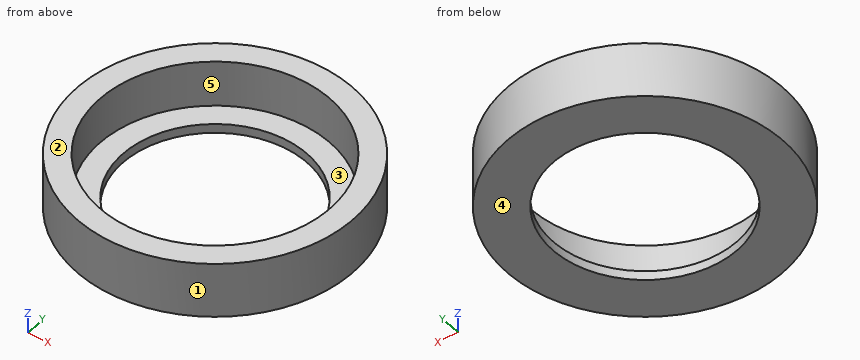
```python
from build123d import *

# Parameters (mm, degrees)
SKETCH_R        = 15
PAD_DEPTH       = 6
SKETCH001_R     = 12.5
POCKET_DEPTH    = 5
SKETCH002_R     = 10
POCKET001_DEPTH = 1.001


with BuildPart() as part:
    # Sketch → Pad (new body)
    with BuildSketch(Plane.XY):
        Circle(SKETCH_R)
    extrude(amount=PAD_DEPTH)

    # Sketch001 (on Face3 of Pad) → Pocket (cut)
    with BuildSketch(Plane.XY.offset(6)):
        Circle(SKETCH001_R)
    extrude(amount=-POCKET_DEPTH, mode=Mode.SUBTRACT)

    # Sketch002 (on Face5 of Pocket) → Pocket001 (cut, through all)
    with BuildSketch(Plane.XY.offset(1)):
        Circle(SKETCH002_R)
    extrude(amount=-POCKET001_DEPTH, mode=Mode.SUBTRACT)


solid = part.part
```
Geometry check sheet. Reference: the model listing, model coordinates, mm. Face numbers are marked on the shaded views. A direction names the side the tool comes from. Coordinates: 2 decimals unless noted, no trailing zeros. Order: outer loops, then holes, each group sorted by start corner. A loop starts at its lowest first (then second) coordinate and runs counter-clockwise, first axis right, second up.
Item 1: Depth check by flat-ended pin: pin 1 (2 mm diameter, centred on y = -5, z = 3, fed in from +X); pin 2 (1 mm diameter, centred on x = 6, z = 1, fed in from +Y); pin 3 (7.5 mm diameter, centred on x = 5.5, y = -5.5, fed in from +Z). Enter the tip coordinate at first touch or a pass-through.
Item 2: Tool access check on the marked faces 4 and 5. Record the directions out of +Z, -Z, +X, -X, +Y, -Y that give a thin tool (end or side, any length) a straight path to the whole face; none if there is none.
Item 3: Section check C-C (z = 0.5). Enter the section's corners in (x, y).
Item 4: Section check A-A (x = 0). Enter the section's corners in (y, z), plus the area to 3 significant figures.
Item 5: Scan lines: line 1 along Y through (x, z) = (0, 0.2); line 2 along Y through (x, z) = (0, 2). Record each from-to range of solid material in increasing order.
Item 6: Section check D-D (y = 11.75). Enter the section's corners in (x, z), plus the area to 3 significant figures.
Item 7: Mould release check, pull along Y, two halves, no side actions. Record for the marked faces 1, 2 and 3: released by +Y, released by -Y, zero draft, split by the parting line, or undercut.
Check sheet entries:
1. pin 1: stops at x = 14.46
1. pin 2: stops at y = 13.96
1. pin 3: stops at z = 1
2. face 4: -Z, +X, -X, +Y, -Y
2. face 5: +Z
3. outline: circle Ø30 at (0, 0); hole circle Ø20 at (0, 0)
4. outline: (-15, 0) - (-10, 0) - (-10, 1) - (-12.5, 1) - (-12.5, 6) - (-15, 6) - close; (10, 0) - (15, 0) - (15, 6) - (12.5, 6) - (12.5, 1) - (10, 1) - close
4. area: 35.0 mm2
5. line 1: y = -15 to -10, 10 to 15
5. line 2: y = -15 to -12.5, 12.5 to 15
6. outline: (-9.32, 0) - (9.32, 0) - (9.32, 6) - (4.26, 6) - (4.26, 1) - (-4.26, 1) - (-4.26, 6) - (-9.32, 6) - close
6. area: 69.2 mm2
7. face 1: split by the parting line
7. face 2: zero draft
7. face 3: undercut
